For this review, take the finished solid that the model builds, in its own axes (mm). A direction names the side the tool comes from. Coordinates: 2 decimals unless noted, no trailing zeros. Order: outer loops, then holes, each group sorted by start corner. A loop starts at its lowest first (then second) coordinate and runs counter-clockwise, first axis right, second up. Notation, with made-up numbers: M 10,13.25 L 67,13.25 A30 cw 67,45.25 Z; hole C 39,15 d10. An arc over 180 degrees is marked long. Use CSV: the item, a comma, the result in double quotes.
```python
from build123d import *

# Parameters (mm, degrees)
CUT_EXTRUDE1_DEPTH      = 14.285330256
CUT_EXTRUDE1_DEPTH_BACK = 14.285330256
SKETCH4_R               = 2
CUT_EXTRUDE2_DEPTH      = 14.285330429
CUT_EXTRUDE2_DEPTH_BACK = 14.285330429
SKETCH5_R               = 2
CUT_EXTRUDE3_DEPTH      = 1.4
CUT_EXTRUDE4_DEPTH      = 1.4
CUT_EXTRUDE5_DEPTH      = 1.4
CUT_EXTRUDE6_DEPTH      = 1.4


with BuildPart() as part:
    # Sketch2 → Revolve1 (revolve)
    with BuildSketch(Plane(origin=(0, 0, 0), x_dir=(0, 0, -1), z_dir=(1, 0, 0)), mode=Mode.PRIVATE) as revolve1_sk:
        Polygon((8, 2.25), (0, 2.25), (0, 3.25), (-8, 3.25), (-8, 7.5), (8, 7.5), align=None)
    revolve(revolve1_sk.sketch.rotate(Axis((0, 0, 33.32637001), (0, 0, -1)), 90), axis=Axis((0, 0, 33.32637001), (0, 0, -1)))

    # Sketch4 → Cut-Extrude1 (cut, two sides: drawn at the far end of the back side and taken through both)
    with BuildSketch(Plane(origin=(0, 0, 0), x_dir=(1, 0, 0), z_dir=(0, 1, 0)).offset(-CUT_EXTRUDE1_DEPTH_BACK)):
        with Locations(Location((0, 4, 0), (0, 0, 270))):
            Circle(SKETCH4_R)
    extrude(amount=CUT_EXTRUDE1_DEPTH + CUT_EXTRUDE1_DEPTH_BACK, mode=Mode.SUBTRACT)

    # Sketch5 → Cut-Extrude2 (cut, two sides: drawn at the far end of the back side and taken through both)
    with BuildSketch(Plane(origin=(0, 0, 0), x_dir=(0, 0, -1), z_dir=(1, 0, 0)).offset(-CUT_EXTRUDE2_DEPTH_BACK)):
        with Locations((-4, 0)):
            Circle(SKETCH5_R)
    extrude(amount=CUT_EXTRUDE2_DEPTH + CUT_EXTRUDE2_DEPTH_BACK, mode=Mode.SUBTRACT)

    # Sketch6 → Cut-Extrude3 (cut, symmetric)
    with BuildSketch(Plane(origin=(4.9, 0, 0), x_dir=(0, 0, -1), z_dir=(1, 0, 0))):
        Polygon((-5.732050808, 3), (-8, 3), (-8, -3), (-5.732050808, -3), (-2.267949192, -3), (-0.535898385, 0), (-2.267949192, 3), align=None)
    extrude(amount=CUT_EXTRUDE3_DEPTH, both=True, mode=Mode.SUBTRACT)

    # Sketch7 → Cut-Extrude4 (cut, symmetric)
    with BuildSketch(Plane(origin=(-4.9, 0, 0), x_dir=(0, 0, -1), z_dir=(1, 0, 0))):
        Polygon((-5.732050808, 3), (-8, 3), (-8, -3), (-5.732050808, -3), (-2.267949192, -3), (-0.535898385, 0), (-2.267949192, 3), align=None)
    extrude(amount=CUT_EXTRUDE4_DEPTH, both=True, mode=Mode.SUBTRACT)

    # Sketch8 → Cut-Extrude5 (cut, symmetric)
    with BuildSketch(Plane(origin=(0, 4, 0), x_dir=(-1, 0, 0), z_dir=(0, 1, 0))):
        Polygon((3, -5.732050808), (3, -8), (-3, -8), (-3, -5.732050808), (-3, -2.267949192), (0, -0.535898385), (3, -2.267949192), align=None)
    extrude(amount=CUT_EXTRUDE5_DEPTH, both=True, mode=Mode.SUBTRACT)

    # Sketch9 → Cut-Extrude6 (cut, symmetric)
    with BuildSketch(Plane(origin=(0, -4, 0), x_dir=(-1, 0, 0), z_dir=(0, 1, 0))):
        Polygon((-3, -5.732050808), (-3, -8), (3, -8), (3, -5.732050808), (3, -2.267949192), (0, -0.535898385), (-3, -2.267949192), align=None)
    extrude(amount=CUT_EXTRUDE6_DEPTH, both=True, mode=Mode.SUBTRACT)


solid = part.part
```
Item 1: Draft analysis for pull direction X (two halves, no side actions). For faces 4 (the face through (1, -5.4, -6)), 5 (the face through (2, -2, -8)), state which applies: released by +X, released by -X, zero draft, split by the parting line, or undercut.
Solutions:
face 4,"undercut"
face 5,"zero draft"
Item 2: Add section C-C on x = 6. State the section outline as (y, z) points, and give its area (3 significant figures).
Solutions:
outline,"M -4.5,-8 L 4.5,-8 L 4.5,8 L 3,8 L 3,2.27 L 0,0.54 L -3,2.27 L -3,8 L -4.5,8 Z"
area,"104 mm^2"
Item 3: For faces 1 (the face through (3.5, 1, 6)), 2 (the face through (1, -2.6, -6)), 3 (the face through (-6.775, -0.766, 2.153)), list the 3-axis set-ups (+Z, -Z, +X, -X, +Y, -Y) from which the entire face can be reached by the end or side of a thin tool; tool diameter is ignored.
Solutions:
face 1,"+Z"
face 2,"-Z"
face 3,"+X, -X"
Item 4: To check wall thickness, follow line 1 along Z through (x, y) = (0, -6.3); line 2 along Y through (x, z) = (2.5, -6.25); line 3 along Z through (x, y) = (-6.85, 0). State the ranges of each line that lie inside material, in increasing order. Write a range as [from, to].
Solutions:
line 1,"[-8, -6], [-2, 8]"
line 2,"[-7.07, -5.4], [-2.6, 2.6], [5.4, 7.07]"
line 3,"[-8, 2], [6, 8]"
Item 5: Add section B-B on z = 1.5. State the section outline as (x, y) points.
Solutions:
outline,"C 0,0 d15; hole M -6.3,-1.67 L -3.5,-1.67 L -3.5,1.67 L -6.3,1.67 Z; hole C 0,0 d6.5; hole M 3.5,-1.67 L 6.3,-1.67 L 6.3,1.67 L 3.5,1.67 Z"
Item 6: Add section D-D on x = -1.75. State how many separate pieces and enclosed holes the cut face has, and give its area (3 significant figures).
Solutions:
separate pieces,"6"
enclosed holes,"0"
area,"119 mm^2"
Item 7: Clearance check with flat-ended pins moving along their axes: pin 1 Ø2 at (y, z) = (1.5, -4.5) entering from -X; pin 2 Ø2 at (y, z) = (-5, 4) entering from +X; pin 3 Ø1.4 at (y, z) = (-4, -6) entering from +X (3 decimals); pin 4 Ø3.5 at (y, z) = (0, 4) entering from +X. State where each tip first meets the part, or that it passes through.
Solutions:
pin 1,"x = -7.48"
pin 2,"x = 6.34"
pin 3,"x = 6.735"
pin 4,"through"
Item 8: Add section A-A on z = 4. State the section outline as (x, y) points, and give its area (3 significant figures).
Solutions:
outline,"M -7.23,-2 A7.5 ccw 7.23,-2 L 6.3,-2 L 6.3,-3 L 3.5,-3 L 3.5,-2 L 2.56,-2 A3.25 cw -2.56,-2 L -3.5,-2 L -3.5,-3 L -6.3,-3 L -6.3,-2 Z; M -7.23,2 L -6.3,2 L -6.3,3 L -3.5,3 L -3.5,2 L -2.56,2 A3.25 cw 2.56,2 L 3.5,2 L 3.5,3 L 6.3,3 L 6.3,2 L 7.23,2 A7.5 ccw Z"
area,"97.3 mm^2"
